from build123d import *

# Parameters (mm, degrees)
FILLET1_R      = 0.3
CHAMFER1_SIZE  = 0.6
CHAMFER1_SIZE2 = 0.346410162
CHAMFER2_SIZE  = 0.5
CHAMFER2_SIZE2 = 0.288675135


with BuildPart() as part:
    # Sketch1 → Revolve1 (revolve)
    with BuildSketch(Plane.XY):
        Polygon((2.45, 0), (4.45, 0), (4.45, -0.9), (2.95, -0.9), (2.95, -11), (2, -11), (2, -4.9), (2.45, -4.9), align=None)
    revolve(axis=Axis((0, 0, 0), (0, -1, 0)))

    # Fillet1
    fillet1_edges = [part.edges().sort_by_distance(p)[0] for p in [
        (-4.45, -0.9, 0),
        (-4.45, 0, 0),
        (-2.45, 0, 0),
    ]]
    fillet(fillet1_edges, radius=FILLET1_R)

    # Chamfer1
    chamfer1_edges = [part.edges().sort_by_distance(p)[0] for p in [
        (-2.95, -11, 0),
    ]]
    chamfer1_side = [part.faces().sort_by_distance(p)[0] for p in [
        (-2.95, -5.95, 0),
    ]]
    chamfer(chamfer1_edges, length=CHAMFER1_SIZE, length2=CHAMFER1_SIZE2, reference=chamfer1_side[0])

    # Chamfer2
    chamfer2_edges = [part.edges().sort_by_distance(p)[0] for p in [
        (-2, -11, 0),
    ]]
    chamfer2_side = [part.faces().sort_by_distance(p)[0] for p in [
        (-2, -7.95, 0),
    ]]
    chamfer(chamfer2_edges, length=CHAMFER2_SIZE, length2=CHAMFER2_SIZE2, reference=chamfer2_side[0])


solid = part.part
Verification items for the finished model (mm, model axes). A direction names the side the tool comes from. Coordinates: 2 decimals unless noted, no trailing zeros. Order: outer loops, then holes, each group sorted by start corner. A loop starts at its lowest first (then second) coordinate and runs counter-clockwise, first axis right, second up.
1. Sectioned sample at B-B, the plane z = 0. Record the cut outline in (x, y), and give its area (3 significant figures).
Results found:
outline: (-4.45, -0.6) arc R0.3 ccw to (-4.15, -0.9) - (-2.95, -0.9) - (-2.95, -10.4) - (-2.6, -11) - (-2.29, -11) - (-2, -10.5) - (-2, -4.9) - (-2.45, -4.9) - (-2.45, -0.3) arc R0.3 ccw to (-2.75, 0) - (-4.15, 0) arc R0.3 ccw to (-4.45, -0.3) - close; (2, -10.5) - (2.29, -11) - (2.6, -11) - (2.95, -10.4) - (2.95, -0.9) - (4.15, -0.9) arc R0.3 ccw to (4.45, -0.6) - (4.45, -0.3) arc R0.3 ccw to (4.15, 0) - (2.75, 0) arc R0.3 ccw to (2.45, -0.3) - (2.45, -4.9) - (2, -4.9) - close
area: 18.7 mm2
2. Sectioned sample at A-A, the plane x = 0. Record the cut outline in (y, z).
Results found:
outline: (-11, -2.6) - (-10.4, -2.95) - (-0.9, -2.95) - (-0.9, -4.15) arc R0.3 ccw to (-0.6, -4.45) - (-0.3, -4.45) arc R0.3 ccw to (0, -4.15) - (0, -2.75) arc R0.3 ccw to (-0.3, -2.45) - (-4.9, -2.45) - (-4.9, -2) - (-10.5, -2) - (-11, -2.29) - close; (-11, 2.29) - (-10.5, 2) - (-4.9, 2) - (-4.9, 2.45) - (-0.3, 2.45) arc R0.3 ccw to (0, 2.75) - (0, 4.15) arc R0.3 ccw to (-0.3, 4.45) - (-0.6, 4.45) arc R0.3 ccw to (-0.9, 4.15) - (-0.9, 2.95) - (-10.4, 2.95) - (-11, 2.6) - close
3. Release check for a two-part mould opening along Z. For faces 1 (the face through (-1, 0, -3)), 2 (the face through (1, -4.9, -2)), 3 (the face through (0, -8, -2)), 4 (the face through (-3.28, -0.45, 3.01)) record: +Z half, -Z half, draft (parallel to the pull), parting line (faces both ways), or undercut.
Results found:
face 1: draft
face 2: undercut
face 3: undercut
face 4: parting line
4. Scan lines: line 1 (Z direction, x = 0, y = -2.05); line 2 (Z direction, x = 0, y = -7); line 3 (Y direction, x = 2.75, z = -1.75). Record each from-to range of solid material in increasing order.
Results found:
line 1: z = -2.95 to -2.45, 2.45 to 2.95
line 2: z = -2.95 to -2, 2 to 2.95
line 3: y = -0.9 to 0
5. Set-up check for faces 5 (the face through (-0.5, -2.6, -2.4)), 6 (the face through (-2.947, -5.717, 0.13)): record each of +Z, -Z, +X, -X, +Y, -Y from which the full face is reachable in a straight line by a thin tool's end or side.
Results found:
face 5: +Y
face 6: -Y
6. Sectioned sample at C-C, the plane y = -5.5. Record the cut outline in (x, z), and give its area (3 significant figures).
Results found:
outline: circle Ø5.9 at (0, 0); hole circle Ø4 at (0, 0)
area: 14.8 mm2
7. Go/stop test with flat-tipped pins: pin 1 Ø2.5 at (x, z) = (0, 0) entering from +Y; pin 2 Ø4 at (x, z) = (1, -3) entering from +Y; pin 3 Ø1.5 at (y, z) = (-9.5, 2) entering from -X. Record where each tip stops, or that it passes through.
Results found:
pin 1: passes through
pin 2: stops at y = 0
pin 3: stops at x = -2.67
